from build123d import *

# Parameters (mm, degrees)
BOSS_EXTRUDE1_DEPTH        = 2
FILLET1_R                  = 15
FILLET3_R                  = 2
M3_CLEARANCE_HOLE1_D       = 3.6
SKETCH7_R                  = 4
BOSS_EXTRUDE2_DEPTH        = 4
F_4_2_4_2_DIAMETER_HOLE1_D = 4.2


with BuildPart() as part:
    # Sketch1 → Boss-Extrude1 (new body)
    with BuildSketch(Plane.XY):
        with BuildLine():
            Line((-10.770329614, -28), (-20, -28))
            Line((-20, -28), (-20, -50))
            Line((-20, -50), (20, -50))
            Line((20, -50), (20, -28))
            Line((20, -28), (10.770329614, -28))
            ThreePointArc((10.770329614, -28), (24.729636961, -16.983670268), (30, 0))
            Line((30, 0), (21, 0))
            ThreePointArc((21, 0), (0, -21), (-21, 0))
            Line((-21, 0), (-30, 0))
            ThreePointArc((-30, 0), (-24.729636961, -16.983670268), (-10.770329614, -28))
        make_face()
    extrude(amount=BOSS_EXTRUDE1_DEPTH)

    # Fillet1
    # the kernel refuses this fillet: 15 mm, written as the material it adds along each edge
    with BuildSketch(Plane(origin=(-10.770329614, -28, 0), x_dir=(-0.8085477056225583, 0.588430631198357, 0), z_dir=(0, 0, 1))) as fillet1_piece_1:
        with BuildLine():
            CenterArc((19.419330938, 14.488463805), FILLET1_R, 217.144663105, 37.84908673)
            Line((7.462628814, 5.431020771), (0, 0))
            ThreePointArc((0, 0), (7.767732375, 1.023072389), (15.53546475, 0))
        make_face()
    extrude(amount=2)
    with BuildSketch(Plane(origin=(10.770329614, -28, 0), x_dir=(0.8085477056225584, 0.5884306311983569, 0), z_dir=(0, 0, 1))) as fillet1_piece_2:
        with BuildLine():
            CenterArc((19.419330938, -14.488463805), FILLET1_R, 105.006250165, 37.84908673)
            Line((7.462628814, -5.431020771), (0, 0))
            ThreePointArc((0, 0), (7.767732375, -1.023072389), (15.53546475, 0))
        make_face()
    extrude(amount=2)

    # Fillet3
    fillet3_edges = [part.edges().sort_by_distance(p)[0] for p in [
        (20, -50, 1),
        (-20, -50, 1),
        (-30, 0, 1),
        (-21, 0, 1),
        (21, 0, 1),
        (30, 0, 1),
    ]]
    fillet(fillet3_edges, radius=FILLET3_R)

    # M3 Clearance Hole1 (through all)
    with Locations(Plane.XY.offset(2)):
        with Locations((10, -30), (-24.620193825, -4.341204442), (-10, -30), (24.620193825, -4.341204442)):
            Hole(M3_CLEARANCE_HOLE1_D / 2)

    # Sketch7 → Boss-Extrude2 (add)
    with BuildSketch(Plane.XY.offset(2)):
        with Locations((-15, -45)):
            Circle(SKETCH7_R)
        with Locations((15, -45)):
            Circle(SKETCH7_R)
        with Locations((15, -23)):
            Circle(SKETCH7_R)
        with Locations((-15, -23)):
            Circle(SKETCH7_R)
    extrude(amount=BOSS_EXTRUDE2_DEPTH)

    # Ø4.2 (4.2) Diameter Hole1 (through all)
    with Locations(Plane.XY.offset(6)):
        with Locations((-15, -23), (15, -23), (15, -45), (-15, -45)):
            Hole(F_4_2_4_2_DIAMETER_HOLE1_D / 2)


solid = part.part
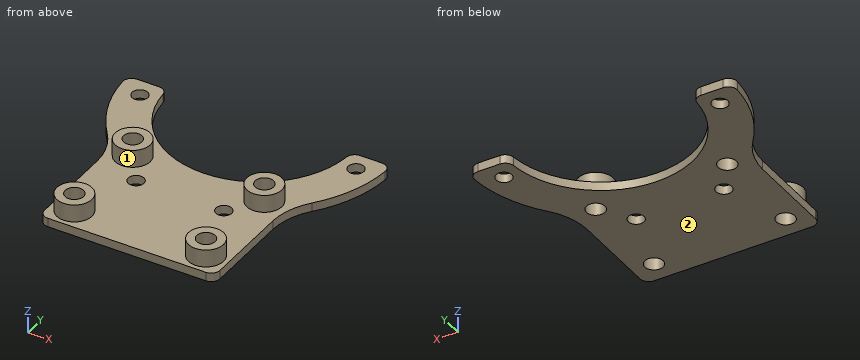
Work out the finished part from the listing and answer in its coordinate system (mm). Face numbers are marked on the shaded views. Round coordinates to 2 decimals unless told otherwise and drop trailing zeros. Write each loop counter-clockwise with the first axis right and the second up, starting at its lowest first coordinate (ties: lowest second). Pieces come first, ordered by that corner, then holes. Notation, with made-up numbers: (3.5, 24) - (31.5, 24) arc R17 cw to (31.5, 50) - close; hole circle Ø4 at (84.25, 84.5). An arc over 180 degrees is marked (long way). Answer in a Markdown table with one row per item. Add a question column.
1. A cutting plane is placed at C-C, the plane x = -10. Determine the outline of the cut face in (y, z), and give its area (3 significant figures).
2. A cutting plane is placed at A-A, the plane y = -30. Determine the outline of the cut face in (x, z), and give its area (3 significant figures).
3. A cutting plane is placed at D-D, the plane y = -45. Determine the outline of the cut face in (x, z).
4. The mould has two halves that part along Y. Classify the marked faces 1 and 2: +Y half, -Y half, draft (parallel to the pull), parting line (faces both ways), or undercut.
5. Given pin 1 (1.5 mm diameter, centred on x = -12, y = -33, fed in from +Z); pin 2 (1 mm diameter, centred on x = -16, z = 5, fed in from -Y); pin 3 (1.6 mm diameter, centred on y = -36.5, z = 0.5, fed in from +X), each flat-ended and moving along its own axis, determine where each tip first touches the part or whether it passes through.
6. A cutting plane is placed at B-B, the plane z = 3. Determine the outline of the cut face in (x, y), and give its area (3 significant figures).
7. Find the intervals of material crossed by line 1 along Y through (x, z) = (-15, 3.05); line 2 along X through (y, z) = (-46.5, 1.7); line 3 along X through (y, z) = (-29, 1.55), in increasing order. Write a range as from..to.
Worked out:
| question | item | result |
|---|---|---|
| 1 | outline | (-50, 0) - (-31.8, 0) - (-31.8, 2) - (-50, 2) - close; (-28.2, 0) - (-18.47, 0) - (-18.47, 2) - (-28.2, 2) - close |
| 1 | area | 55.9 mm^2 |
| 2 | outline | (-20, 0) - (-11.8, 0) - (-11.8, 2) - (-20, 2) - close; (-8.2, 0) - (8.2, 0) - (8.2, 2) - (-8.2, 2) - close; (11.8, 0) - (20, 0) - (20, 2) - (11.8, 2) - close |
| 2 | area | 65.6 mm^2 |
| 3 | outline | (-20, 0) - (-17.1, 0) - (-17.1, 6) - (-19, 6) - (-19, 2) - (-20, 2) - close; (-12.9, 0) - (12.9, 0) - (12.9, 6) - (11, 6) - (11, 2) - (-11, 2) - (-11, 6) - (-12.9, 6) - close; (17.1, 0) - (20, 0) - (20, 2) - (19, 2) - (19, 6) - (17.1, 6) - close |
| 4 | face 1 | undercut |
| 4 | face 2 | draft |
| 5 | pin 1 | z = 2 |
| 5 | pin 2 | y = -48.97 |
| 5 | pin 3 | x = 20 |
| 6 | outline | circle Ø8 at (-15, -45); circle Ø8 at (-15, -23); circle Ø8 at (15, -45); circle Ø8 at (15, -23); hole circle Ø4.2 at (-15, -45); hole circle Ø4.2 at (-15, -23); hole circle Ø4.2 at (15, -45); hole circle Ø4.2 at (15, -23) |
| 6 | area | 146 mm^2 |
| 7 | line 1 | -49..-47.1, -42.9..-41, -27..-25.1, -20.9..-19 |
| 7 | line 2 | -20..-16.47, -13.53..13.53, 16.47..20 |
| 7 | line 3 | -20..-11.5, -8.5..8.5, 11.5..20 |
